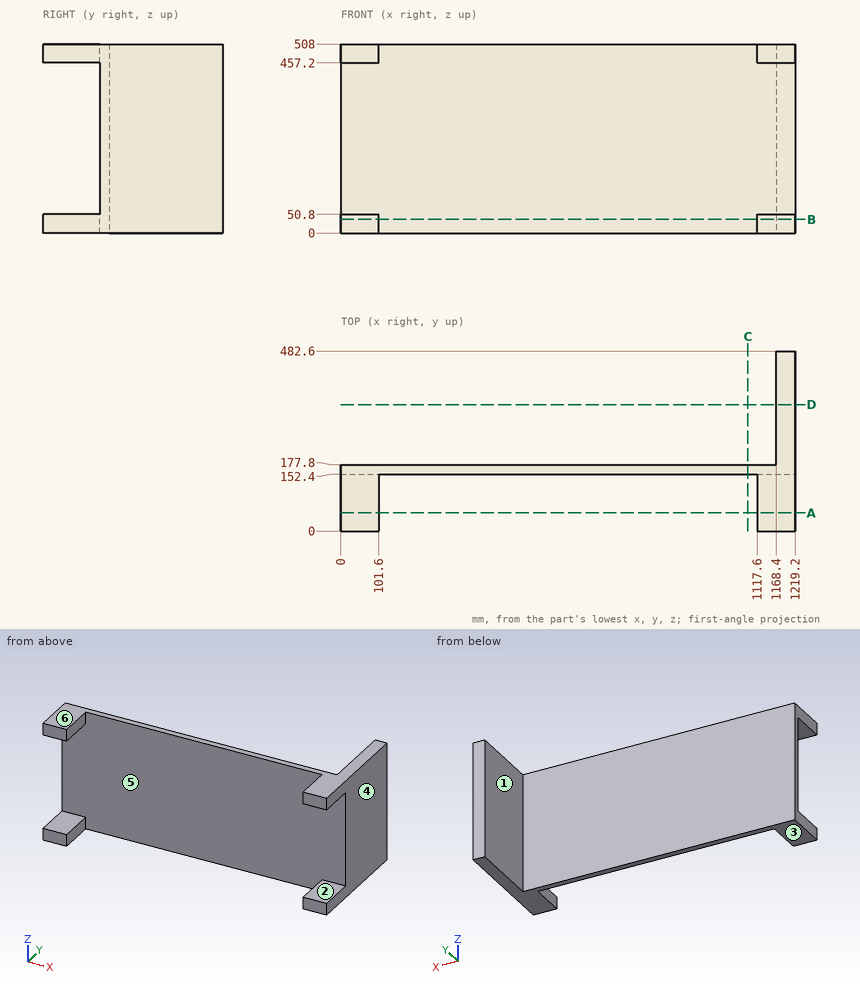
Source: three-view drawing plus pictorial views. Frame: mm from the lowest corner of the part. A direction names the side the tool comes from. Give positions to 0.01 mm unless a question says otherwise; leave off trailing zeros. Write each loop counter-clockwise with the first axis right and the second up, starting at its lowest first coordinate (ties: lowest second). Pieces come first, ordered by that corner, then holes.
(1) Cut plane C-C, the plane x = 1092.5. Return loops of the section in (y, z), then the cut area to 3 significant figures.
(2) Cut plane B-B, the plane z = 37. Return loops of the section in (x, y), then the cut area to 3 significant figures.
(3) Access query for the marked faces 1, 2 and 3. Directions: +Z, -Z, +X, -X, +Y, -Y. A direction counts if a zero-diameter tool reaches every point of the face in a straight line with its end or side. Return the directions, or none.
(4) Cut plane A-A, the plane y = 48.5. Return loops of the section in (x, z).
(5) Mould query, pull axis Z, two halves, no side actions, for the marked faces 4, 5 and 6. Classes: released by +Z, released by -Z, zero draft, split by the parting line, or undercut.
(6) Ray query, line 1 (X direction, y = 53, z = 484); line 2 (X direction, y = 248, z = 218.5); line 3 (Y direction, x = 240, z = 386.5). Return the intervals inside material, ascending.
(7) Cut plane D-D, the plane y = 339. Return loops of the section in (x, z), then the cut area to 3 significant figures.
(8) First-contact query: P1, Ø5, axis at y = 364.5, z = 179, coming from the -X side; P2, Ø1, axis at x = 382, z = 88, coming from the +Y side. Flat tips, straight axial feed; report the tip coordinate or a pass-through.
Values follow:
1. outline: (152.4, 0) - (177.8, 0) - (177.8, 508) - (152.4, 508) - close
1. area: 12,900 mm2
2. outline: (0, 0) - (101.6, 0) - (101.6, 152.4) - (1117.6, 152.4) - (1117.6, 0) - (1219.2, 0) - (1219.2, 482.6) - (1168.4, 482.6) - (1168.4, 177.8) - (0, 177.8) - close
2. area: 77,400 mm2
3. face 1: +Z, -Z, -X, +Y
3. face 2: +X, -X, -Y
3. face 3: -Z, +X, -X, +Y, -Y
4. outline: (0, 0) - (101.6, 0) - (101.6, 50.8) - (0, 50.8) - close; (0, 457.2) - (101.6, 457.2) - (101.6, 508) - (0, 508) - close; (1117.6, 0) - (1219.2, 0) - (1219.2, 50.8) - (1117.6, 50.8) - close; (1117.6, 457.2) - (1219.2, 457.2) - (1219.2, 508) - (1117.6, 508) - close
5. face 4: zero draft
5. face 5: undercut
5. face 6: released by +Z
6. line 1: x = 0 to 101.6, 1117.6 to 1219.2
6. line 2: x = 1168.4 to 1219.2
6. line 3: y = 152.4 to 177.8
7. outline: (1168.4, 0) - (1219.2, 0) - (1219.2, 508) - (1168.4, 508) - close
7. area: 25,800 mm2
8. P1: stops at x = 1168.4
8. P2: stops at y = 177.8
